from build123d import *

# Parameters (mm, degrees)
SKETCH1_R             = 4
SKETCH1_R_2           = 2.5
BOSS_EXTRUDE1_DEPTH   = 10
BOSS_EXTRUDE1_2_DEPTH = 10
BOSS_EXTRUDE1_3_DEPTH = 10
SKETCH2_W             = 15
SKETCH2_H             = 30
BOSS_EXTRUDE2_DEPTH   = 2
CUT_EXTRUDE1_START    = -2
SKETCH3_R             = 2.5
CUT_EXTRUDE1_DEPTH    = 2
CUT_EXTRUDE3_DEPTH    = 22
FILLET2_R             = 2


with BuildPart() as part:
    # Sketch1 → Boss-Extrude1 (new body)
    with BuildSketch(Plane.XY):
        with Locations((-0.039690435, 8.999912481)):
            Circle(SKETCH1_R)
        with Locations((-0.039690435, 8.999912481)):
            Circle(SKETCH1_R_2, mode=Mode.SUBTRACT)
    extrude(amount=BOSS_EXTRUDE1_DEPTH)



with BuildPart() as body_2:
    # Sketch1 → Boss-Extrude1 2 (new body)
    with BuildSketch(Plane.XY):
        Circle(SKETCH1_R)
        Circle(SKETCH1_R_2, mode=Mode.SUBTRACT)
    extrude(amount=BOSS_EXTRUDE1_2_DEPTH)


with BuildPart() as body_3:
    # Sketch1 → Boss-Extrude1 3 (new body)
    with BuildSketch(Plane.XY):
        with Locations((-0.039620931, -8.999912787)):
            Circle(SKETCH1_R)
        with Locations((-0.039620931, -8.999912787)):
            Circle(SKETCH1_R_2, mode=Mode.SUBTRACT)
    extrude(amount=BOSS_EXTRUDE1_3_DEPTH)


with BuildPart() as part_1:
    add(part.part)

    add(body_2.part)  # Boss-Extrude2 merges body 2

    add(body_3.part)  # Boss-Extrude2 merges body 3
    # Sketch2 → Boss-Extrude2 (add)
    with BuildSketch(Plane(origin=(0, 0, 0), x_dir=(-1, 0, 0), z_dir=(0, 0, -1))):
        Rectangle(SKETCH2_W, SKETCH2_H)
    extrude(amount=BOSS_EXTRUDE2_DEPTH)

    # Sketch3 → Cut-Extrude1 (cut)
    with BuildSketch(Plane.XY.offset(CUT_EXTRUDE1_START)):
        with Locations((-0.039690435, 8.999912481)):
            Circle(SKETCH3_R)
        Circle(SKETCH3_R)
        with Locations((-0.039620931, -8.999912787)):
            Circle(SKETCH3_R)
    extrude(amount=CUT_EXTRUDE1_DEPTH, mode=Mode.SUBTRACT)

    # Sketch4 → Cut-Extrude3 (cut)
    with BuildSketch(Plane.ZY.offset(7.5)):
        Polygon((10, 4.000087213), (10, -3.999912787), (10, -4.510778231), (3, -4.510778231), (3, -3.999912787), align=None)
        Polygon((10, 13.000087213), (10, 5.000087213), (10, 4.572676738), (3, 4.572676738), (3, 5.000087213), align=None)
        Polygon((10, -4.999912787), (10, -12.999912787), (10, -13.831411627), (3, -13.831411627), (3, -12.999912787), align=None)
    extrude(amount=-CUT_EXTRUDE3_DEPTH, mode=Mode.SUBTRACT)

    # Fillet2
    fillet2_edges = [part_1.edges().sort_by_distance(p)[0] for p in [
        (7.5, -15, -1),
        (-7.5, -15, -1),
        (-7.5, 15, -1),
        (7.5, 15, -1),
    ]]
    fillet(fillet2_edges, radius=FILLET2_R)


solid = part_1.part
Can you work these out from the model? Positions are in its coordinate system, mm. A direction names the side the tool comes from. Give positions to 0.01 mm unless a question says otherwise; leave off trailing zeros. Loops run counter-clockwise (first coordinate to the right, second up) from the corner with the lowest first, then second, coordinate; pieces in that order, holes last. Notation, with made-up numbers: (-9, 85.5) -> (12, 85.5) arc R8 cw to (12, 91.5) -> close; hole circle Ø5 at (23.25, 8.25). An arc over 180 degrees is marked (long way). Return JSON: item names as keys, results as strings.
Q1. For pin 1 Ø5 at (x, z) = (3.5, 3) entering from +Y; pin 2 Ø8 at (x, y) = (1.5, -12) entering from +Z; pin 3 Ø5 at (y, z) = (-4.5, 4.5) entering from -X, each with a flat end and sliding along its axis, tell me the tip position at first contact or that it passes through.
Checks:
{"pin 1": "stops at y = 12.86", "pin 2": "stops at z = 7.31", "pin 3": "stops at x = -3.5"}
Q2. I want a section at C-C, the plane y = -7. List the corners of the cut face in (x, z) for me.
Checks:
{"outline": "(-7.5, -2) -> (-1.54, -2) -> (-1.54, 8.25) -> (-3.5, 8.25) -> (-3.5, 0) -> (-7.5, 0) -> close; (1.46, -2) -> (7.5, -2) -> (7.5, 0) -> (3.42, 0) -> (3.42, 8.25) -> (1.46, 8.25) -> close"}
Q3. On a 3-axis mill with a long thin cutter (end or side, diameter ignored), from which of +Z, -Z, +X, -X, +Y, -Y can I reach the whole of each face in a straight line? I mean faces 1 (the face through (2.6, 9.8, 7.2)), 2 (the face through (6.93, -14.4, -1.01)), 3 (the face through (-0.56, 12.966, 3.819)). Say none if no direction works.
Checks:
{"face 1": "+Z, +X, -X", "face 2": "+Z, -Z, +X, -Y", "face 3": "+Z"}
Q4. I want a section at A-A, the plane z = 3.5. List the corners of the cut face in (x, y) for me.
Checks:
{"outline": "(-2.1, -12.43) -> (2.02, -12.43) arc R4 ccw (long way) to start; (-2.1, 5.57) -> (2.02, 5.57) arc R4 ccw (long way) to start; (-2.06, -3.43) -> (2.06, -3.43) arc R4 ccw (long way) to start; hole circle Ø5 at (-0.04, -9); hole circle Ø5 at (-0.04, 9); hole circle Ø5 at (0, 0)"}
Q5. I need wall thicknesses on probe 1 along Y at (x, z) = (0, 6); probe 2 along Y at (x, z) = (-3.5, 7); probe 3 along X at (y, z) = (0, 4.5). Which ranges of each line are inside material? Lowest first, please.
Checks:
{"probe 1": "y = -6.5 to -5, 2.5 to 4, 11.5 to 13", "probe 2": "y = -8.43 to -6.99, 0.57 to 1.94, 9.57 to 11.01", "probe 3": "x = -4 to -2.5, 2.5 to 4"}
Q6. I want a section at D-D, the plane z = -1. List the corners of the cut face in (x, y) for me, then the cut area to 3 significant figures.
Checks:
{"outline": "(-7.5, -13) arc R2 ccw to (-5.5, -15) -> (5.5, -15) arc R2 ccw to (7.5, -13) -> (7.5, 13) arc R2 ccw to (5.5, 15) -> (-5.5, 15) arc R2 ccw to (-7.5, 13) -> close; hole circle Ø5 at (-0.04, -9); hole circle Ø5 at (-0.04, 9); hole circle Ø5 at (0, 0)", "area": "388 mm2"}
Q7. I want a section at B-B, the plane x = 2. List the corners of the cut face in (y, z) for me, then the cut area to 3 significant figures.
Checks:
{"outline": "(-15, -2) -> (-10.45, -2) -> (-10.45, 5.24) -> (-12.44, 3.49) -> (-12.44, 0) -> (-15, 0) -> close; (-7.55, -2) -> (-1.5, -2) -> (-1.5, 5.19) -> (-3.46, 3.47) -> (-3.46, 0) -> (-5.56, 0) -> (-5.56, 9.51) -> (-7.55, 7.76) -> close; (1.5, -2) -> (7.55, -2) -> (7.55, 5.23) -> (5.56, 3.49) -> (5.56, 0) -> (3.46, 0) -> (3.46, 9.53) -> (1.5, 7.81) -> close; (10.45, -2) -> (15, -2) -> (15, 0) -> (12.44, 0) -> (12.44, 9.51) -> (10.45, 7.76) -> close", "area": "120 mm2"}
